The model under review builds one solid part; all positions refer to its coordinate system, in mm. Face numbers are marked on the shaded views. Coordinates: 2 decimals unless noted, no trailing zeros. Write each loop counter-clockwise with the first axis right and the second up, starting at its lowest first coordinate (ties: lowest second). Pieces come first, ordered by that corner, then holes.
Autodesk Inventor part; units mm, degrees
ref_plane "YZ Plane" through (0, 0, 0) normal (1, 0, 0) x (0, 1, 0)
ref_plane "XZ Plane" through (0, 0, 0) normal (0, 1, 0) x (-1, 0, 0)
ref_plane "XY Plane" through (0, 0, 0) normal (0, 0, 1) x (1, 0, 0)
sketch "スケッチ1" plane through (0, 0, 0) normal (0, 0, 1) x (1, 0, 0)
  circle A0 centre (0, 0) radius 3.5
  circle A1 centre (0, 0) radius 11
  circle A2 centre (0, 0) radius 9.4
  circle A3 centre (0, 0) radius 1.5
  dimension "HUB_DIA" = 7
  dimension "DIA" = 22
  dimension "d5" = 1.6
  dimension "d16" = 3
extrude "ハブ＆リム" add sketch "スケッチ1" along normal blind 8
sketch "スケッチ2" plane through (0, 0, 0) normal (0, 0, 1) x (1, 0, 0)
  line L0 (-0.6, 2.5) -> (0.6, 2.5)
  line L1 (0.6, 2.5) -> (0.6, 10)
  line L2 (0.6, 10) -> (-0.6, 10)
  line L3 (-0.6, 10) -> (-0.6, 2.5)
  line L4 (0, 0) -> (0, 15.4673) construction
  point P0 (0, 2.5)
  dimension "d8" = 2.5
  dimension "d9" = 10
  dimension "d10" = 1.2
extrude "スポーク" add sketch "スケッチ2" along normal blind 8
pattern_circular "円形状パターン1" count 6 over 360 about axis through (0, 0, -10) along (0, 0, 1) of "スポーク"
properties part number "Wheel-D22A"
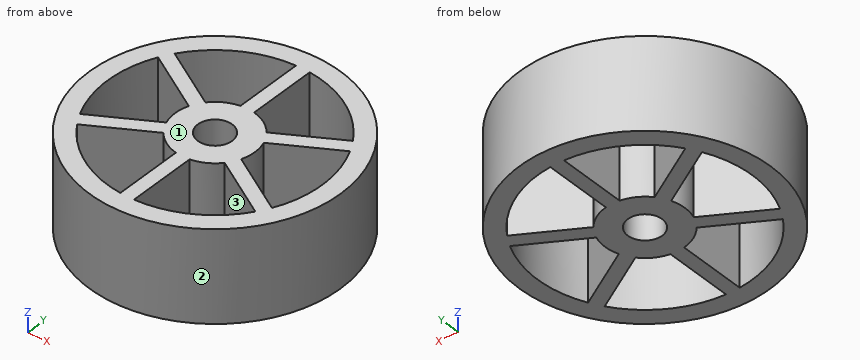
Item 1: For pin 1 (1 mm diameter, centred on x = -7.5, z = 5, fed in from +Y); pin 2 (2 mm diameter, centred on y = 5, z = 4.5, fed in from +X); pin 3 (4.5 mm diameter, centred on y = 7.5, z = 5, fed in from +X), all flat-tipped, find the tip position at first contact; note any pin that passes through.
Solved:
pin 1: stops at y = 8.49
pin 2: stops at x = 10.25
pin 3: stops at x = 9.67
Item 2: Mouldability with a two-part tool opening along Y and no side actions: class the marked faces 1, 2 and 3 as pulls with the +Y half, pulls with the -Y half, needs draft (parallel to the pull), parting line crosses it, or undercut.
Solved:
face 1: needs draft
face 2: parting line crosses it
face 3: undercut
Item 3: Take a section at B-B, the plane x = 0. Write out the cut boundary in (y, z), plus the area to 3 significant figures.
Solved:
outline: (-11, 0) - (-1.5, 0) - (-1.5, 8) - (-11, 8) - close; (1.5, 0) - (11, 0) - (11, 8) - (1.5, 8) - close
area: 152 mm2
Item 4: Take a section at C-C, the plane y = 0. Write out the cut boundary in (x, z), plus the area to 3 significant figures.
Solved:
outline: (-11, 0) - (-9.4, 0) - (-9.4, 8) - (-11, 8) - close; (-3.5, 0) - (-1.5, 0) - (-1.5, 8) - (-3.5, 8) - close; (1.5, 0) - (3.5, 0) - (3.5, 8) - (1.5, 8) - close; (9.4, 0) - (11, 0) - (11, 8) - (9.4, 8) - close
area: 57.6 mm2
Item 5: Take a section at A-A, the plane z = 1.5. Write out the cut boundary in (x, y).
Solved:
outline: circle Ø22 at (0, 0); hole (-8.42, -4.17) - (-3.29, -1.2) arc R3.5 cw to (-3.29, 1.2) - (-8.42, 4.17) arc R9.4 ccw to start; hole (-7.82, -5.21) arc R9.4 ccw to (-0.6, -9.38) - (-0.6, -3.45) arc R3.5 cw to (-2.69, -2.24) - close; hole (-7.82, 5.21) - (-2.69, 2.24) arc R3.5 cw to (-0.6, 3.45) - (-0.6, 9.38) arc R9.4 ccw to start; hole circle Ø3 at (0, 0); hole (0.6, -9.38) arc R9.4 ccw to (7.82, -5.21) - (2.69, -2.24) arc R3.5 cw to (0.6, -3.45) - close; hole (0.6, 3.45) arc R3.5 cw to (2.69, 2.24) - (7.82, 5.21) arc R9.4 ccw to (0.6, 9.38) - close; hole (3.29, -1.2) - (8.42, -4.17) arc R9.4 ccw to (8.42, 4.17) - (3.29, 1.2) arc R3.5 cw to start
Item 6: Take a section at D-D, the plane y = 7.75. Write out the cut boundary in (x, z), plus the area to 3 significant figures.
Solved:
outline: (-7.81, 0) - (-5.32, 0) - (-5.32, 8) - (-7.81, 8) - close; (-0.6, 0) - (0.6, 0) - (0.6, 8) - (-0.6, 8) - close; (5.32, 0) - (7.81, 0) - (7.81, 8) - (5.32, 8) - close
area: 49.4 mm2
Item 7: To check wall thickness, follow line 1 along Y through (x, z) = (0, 2.25); line 2 along Y through (x, z) = (7.5, 4.75); line 3 along X through (y, z) = (5.25, 4). State the ranges of each line that lie inside material, in increasing order.
Solved:
line 1: y = -11 to -1.5, 1.5 to 11
line 2: y = -8.05 to -5.67, -5.02 to -3.64, 3.64 to 5.02, 5.67 to 8.05
line 3: x = -9.67 to -7.8, -0.6 to 0.6, 7.8 to 9.67
